Autodesk Inventor part; units mm, degrees
ref_plane "Work Plane1" through (0, 7, 0) normal (0, -1, 0) x (1, 0, 0)
ref_plane "YZ Plane" through (0, 0, 0) normal (1, 0, 0) x (0, 1, 0)
ref_plane "XZ Plane" through (0, 0, 0) normal (0, 1, 0) x (-1, 0, 0)
sketch "Sketch1" plane through (0, 0, 0) normal (0, 1, 0) x (-1, 0, 0)
  circle A0 centre (0, 0) radius 14
  dimension "d0" = 28
extrude "Extrusion1" add sketch "Sketch1" along normal blind 100
ref_plane "Work Plane1" through (0, 7, 0) normal (0, -1, 0) x (1, 0, 0)
sketch "Sketch2" plane through (0, 7, 0) normal (0, -1, 0) x (1, 0, 0)
  circle A0 centre (0, 0) radius 16
  dimension "d4" = 32
extrude "Extrusion2" add sketch "Sketch2" against normal blind 86
thread "Thread1"
thread "Thread2"
properties part number "Support Tube (Filament Holder" material "ABS Plastic"
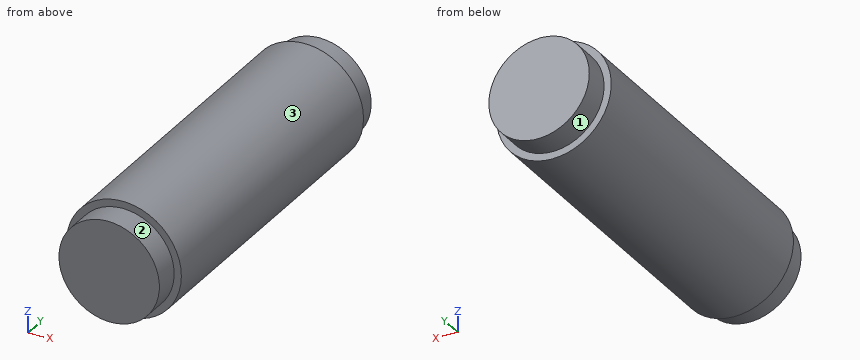
Model file for the job. Use its own axes, mm. Face numbers are marked on the shaded views. A direction names the side the tool comes from. Coordinates: 2 decimals unless noted, no trailing zeros. Loops run counter-clockwise (first coordinate to the right, second up) from the corner with the lowest first, then second, coordinate; pieces in that order, holes last. Notation, with made-up numbers: (-29, 58) - (-21, 58) arc R23 cw to (-21, 82) - close; hole circle Ø8 at (-29, 29). An arc over 180 degrees is marked (long way). Answer as a JSON object with one key per item and string values. Group by question number.
(1) Tool access for the marked faces 1, 2 and 3: list every direction of +Z, -Z, +X, -X, +Y, -Y with a clear straight run to the whole face (end or side of a thin tool).
(2) Cut at B-B (z = 0). Give the cut face in (x, y), then the cut area to 3 significant figures.
(3) Cut at C-C (y = 32.5). Give the cut face in (x, z), then the cut area to 3 significant figures.
(4) Cut at A-A (x = 0). Give the cut face in (y, z), then the cut area to 3 significant figures.
(5) Probe line 1 along X through (y, z) = (54, 12); line 2 along Z through (x, y) = (9, 84); line 3 along X through (y, z) = (63.5, -0.5). List the from-to ranges inside material, lowest first.
(6) Flat gauge pins, fed straight in: pin 1 (8 mm diameter, centred on y = 13.5, z = 5.5, fed in from -X); pin 2 (1 mm diameter, centred on y = 18.5, z = -3.5, fed in from +X); pin 3 (5 mm diameter, centred on x = -12.5, y = 44, fed in from +Z). Where does each tip first touch, or does it go through?
Geometry says:
{
 "1": {"face 1": "+Y", "face 2": "-Y", "face 3": "+Y, -Y"},
 "2": {"outline": "(-16, 7) - (-14, 7) - (-14, 0) - (14, 0) - (14, 7) - (16, 7) - (16, 93) - (14, 93) - (14, 100) - (-14, 100) - (-14, 93) - (-16, 93) - close", "area": "3,140 mm^2"},
 "3": {"outline": "circle Ø32 at (0, 0)", "area": "804 mm^2"},
 "4": {"outline": "(0, -14) - (7, -14) - (7, -16) - (93, -16) - (93, -14) - (100, -14) - (100, 14) - (93, 14) - (93, 16) - (7, 16) - (7, 14) - (0, 14) - close", "area": "3,140 mm^2"},
 "5": {"line 1": "x = -10.58 to 10.58", "line 2": "z = -13.23 to 13.23", "line 3": "x = -15.99 to 15.99"},
 "6": {"pin 1": "stops at x = -15.93", "pin 2": "stops at x = 15.72", "pin 3": "stops at z = 12.49"}
}
